Geometry check sheet. Reference: the model listing, model coordinates, mm. A direction names the side the tool comes from. Give positions to 0.01 mm unless a question says otherwise; leave off trailing zeros. Loops run counter-clockwise (first coordinate to the right, second up) from the corner with the lowest first, then second, coordinate; pieces in that order, holes last. Notation, with made-up numbers: (-10.5, -23.75) -> (8.5, -23.75) arc R13 ccw to (8.5, -6.75) -> close; hole circle Ø1 at (19.25, 6). An arc over 180 degrees is marked (long way). Write item = value, one per line.
```python
from build123d import *

# Parameters (mm, degrees)
BOSS_EXTRUDE1_DEPTH = 20
CUT_EXTRUDE1_REACH  = 33.532
FILLET1_R           = 5
FILLET2_R           = 0.79375


with BuildPart() as part:
    # Sketch1 → Boss-Extrude1 (new, symmetric)
    with BuildSketch(Plane(origin=(0, 0, 0), x_dir=(0, 0, -1), z_dir=(1, 0, 0))):
        Polygon((-4, 0), (10.5, 0), (10.5, 6), (2, 6), (1, 22), (1, 28), (-1, 28), (-1, 22), (-2, 6), (-4, 6), align=None)
    extrude(amount=BOSS_EXTRUDE1_DEPTH, both=True)

    # Sketch4 → Cut-Extrude1 (cut, up to next)
    with BuildSketch(Plane(origin=(0, 6, 0), x_dir=(1, 0, 0), z_dir=(0, 1, 0)), mode=Mode.PRIVATE) as cut_extrude1_sk1:
        with BuildLine():
            Line((-15, 7.55), (-5, 7.55))
            ThreePointArc((-5, 7.55), (-3.45, 6), (-5, 4.45))
            Line((-5, 4.45), (-15, 4.45))
            ThreePointArc((-15, 4.45), (-16.55, 6), (-15, 7.55))
        make_face()
    cut_extrude1_tool1 = extrude(cut_extrude1_sk1.sketch, amount=-CUT_EXTRUDE1_REACH, mode=Mode.PRIVATE) & part.part
    # Sketch4 → Cut-Extrude1 (cut, up to next)
    with BuildSketch(Plane(origin=(0, 6, 0), x_dir=(1, 0, 0), z_dir=(0, 1, 0)), mode=Mode.PRIVATE) as cut_extrude1_sk2:
        with BuildLine():
            Line((5, 7.55), (15, 7.55))
            ThreePointArc((15, 7.55), (16.55, 6), (15, 4.45))
            Line((15, 4.45), (5, 4.45))
            ThreePointArc((5, 4.45), (3.45, 6), (5, 7.55))
        make_face()
    cut_extrude1_tool2 = extrude(cut_extrude1_sk2.sketch, amount=-CUT_EXTRUDE1_REACH, mode=Mode.PRIVATE) & part.part
    add(cut_extrude1_tool1.solids().sort_by_distance((-10, 6, -6))[0], mode=Mode.SUBTRACT)
    add(cut_extrude1_tool2.solids().sort_by_distance((10, 6, -6))[0], mode=Mode.SUBTRACT)

    # Fillet1
    fillet1_edges = [part.edges().sort_by_distance(p)[0] for p in [
        (20, 3, -10.5),
        (-20, 3, -10.5),
    ]]
    fillet(fillet1_edges, radius=FILLET1_R)

    # Fillet2
    fillet2_edges = [part.edges().sort_by_distance(p)[0] for p in [
        (-20, 3, 4),
        (0, 6, 2),
        (0, 22, 1),
        (0, 22, -1),
        (0, 6, -2),
        (20, 3, 4),
    ]]
    fillet(fillet2_edges, radius=FILLET2_R)


solid = part.part
```
Item 1: Tool access check on faces 1 (the cylindrical face through (3.45, 3.04, -5.97)), 2 (the flat face through (0, 6, -7)), 3 (the flat face through (0, 25, 1)). Record the directions out of +Z, -Z, +X, -X, +Y, -Y that give a thin tool (end or side, any length) a straight path to the whole face; none if there is none.
Answer:
face_1 = +Y, -Y
face_2 = -Z, +X, -X, +Y
face_3 = +Z, +X, -X, +Y
Item 2: Gauge pin test, flat ends, axial feed: pin 1 (1.8 mm diameter, centred on x = 4, y = 26, fed in from -Z); pin 2 (1.5 mm diameter, centred on x = 6.5, z = -4, fed in from +Y); pin 3 (2 mm diameter, centred on x = 5.5, y = 24.5, fed in from +Z). Record the tip position at first contact, or that the pin passes through.
Answer:
pin_1 = -1
pin_2 = 6
pin_3 = 1
Item 3: Section check B-B, the plane y = 2. Record the cut outline in (x, z), plus the area to 3 significant figures.
Answer:
outline = (-20, -5.5) arc R5 ccw to (-15, -10.5) -> (15, -10.5) arc R5 ccw to (20, -5.5) -> (20, 3.21) arc R0.79 ccw to (19.21, 4) -> (-19.21, 4) arc R0.79 ccw to (-20, 3.21) -> close; hole (-15, -7.55) -> (-5, -7.55) arc R1.55 ccw to (-5, -4.45) -> (-15, -4.45) arc R1.55 ccw to start; hole (5, -7.55) -> (15, -7.55) arc R1.55 ccw to (15, -4.45) -> (5, -4.45) arc R1.55 ccw to start
area = 492 mm^2
Item 4: Draft check along Z on faces 4 (the flat face through (0, 3, -10.5)), 5 (the flat face through (-10, 3, -7.55)), 6 (the flat face through (0, 6, 3)), 7 (the flat face through (0, 3, 4)). Enter one of: +Z half, -Z half, draft (parallel to the pull), parting line (faces both ways), or undercut.
Answer:
face_4 = -Z half
face_5 = undercut
face_6 = draft
face_7 = +Z half
Item 5: Section check C-C, the plane z = -6. Record the cut outline in (x, y), plus the area to 3 significant figures.
Answer:
outline = (-19.97, 0) -> (-16.55, 0) -> (-16.55, 6) -> (-19.97, 6) -> close; (-3.45, 0) -> (3.45, 0) -> (3.45, 6) -> (-3.45, 6) -> close; (16.55, 0) -> (19.97, 0) -> (19.97, 6) -> (16.55, 6) -> close
area = 82.5 mm^2
Item 6: Section check A-A, the plane x = -6. Record the cut outline in (y, z), plus the area to 3 significant figures.
Answer:
outline = (0, -10.5) -> (6, -10.5) -> (6, -7.55) -> (0, -7.55) -> close; (0, -4.45) -> (6, -4.45) -> (6, -2.75) arc R0.79 cw to (6.74, -1.95) -> (22, -1) -> (28, -1) -> (28, 1) -> (22, 1) -> (6.74, 1.95) arc R0.79 cw to (6, 2.75) -> (6, 4) -> (0, 4) -> close
area = 129 mm^2
Item 7: Thickness scan on L1, parallel to Z at x = -11.5, y = 3.5; L2, parallel to Y at x = 6.5, z = -2.75; L3, parallel to Z at x = 16, y = 3.25. Record the ranges inside material, lowest first. Write a range as [from, to].
Answer:
L1 = [-10.5, -7.55], [-4.45, 4]
L2 = [0, 6]
L3 = [-10.4, -7.18], [-4.82, 4]
Item 8: Section check D-D, the plane x = -17. Record the cut outline in (y, z), plus the area to 3 significant figures.
Answer:
outline = (0, -10.08) -> (6, -10.08) -> (6, -2.75) arc R0.79 cw to (6.74, -1.95) -> (22, -1) -> (28, -1) -> (28, 1) -> (22, 1) -> (6.74, 1.95) arc R0.79 cw to (6, 2.75) -> (6, 4) -> (0, 4) -> close
area = 145 mm^2
